Design review of the part built by this model. Coordinates are the model's own, in mm. A direction names the side the tool comes from. Round coordinates to 2 decimals unless told otherwise and drop trailing zeros. Order: outer loops, then holes, each group sorted by start corner. A loop starts at its lowest first (then second) coordinate and runs counter-clockwise, first axis right, second up.
from build123d import *

# Parameters (mm, degrees)
SKETCH_1_W          = 70
SKETCH_1_H          = 43
EXTRUDE_1_DEPTH     = 10.5
SKETCH_2_R          = 1.5
CUT_EXTRUDE_1_DEPTH = 15
SKETCH_3_W          = 41
SKETCH_3_H          = 20.2
CUT_EXTRUDE_2_DEPTH = 6
SKETCH_4_R          = 7
CUT_EXTRUDE_3_DEPTH = 8.5
SKETCH_6_W          = 39
SKETCH_6_H          = 20.2
CUT_EXTRUDE_4_DEPTH = 2.5
SKETCH_7_R          = 1.525
CUT_EXTRUDE_5_DEPTH = 5
SKETCH_9_W          = 55
SKETCH_9_H          = 1.8
CUT_EXTRUDE_6_DEPTH = 2
FILLET_1_R          = 8
SKETCH_10_R         = 7
SKETCH_10_R_2       = 1.5
SKETCH_10_R_3       = 1.525
CUT_EXTRUDE_7_DEPTH = 20
SKETCH_11_R         = 1.6
CUT_EXTRUDE_8_DEPTH = 1


with BuildPart() as part:
    # 草图1 → 凸台-拉伸1 (new body)
    with BuildSketch(Plane(origin=(0, 0, 0), x_dir=(1, 0, 0), z_dir=(0, 1, 0))):
        with Locations((0, 3.5)):
            Rectangle(SKETCH_1_W, SKETCH_1_H)
    extrude(amount=EXTRUDE_1_DEPTH)

    # 草图2 → 切除-拉伸1 (cut)
    with BuildSketch(Plane(origin=(0, 10.5, 0), x_dir=(1, 0, 0), z_dir=(0, 1, 0))):
        with Locations((15.1, 0)):
            Circle(SKETCH_2_R)
        with Locations((-15.1, 0)):
            Circle(SKETCH_2_R)
    extrude(amount=-CUT_EXTRUDE_1_DEPTH, mode=Mode.SUBTRACT)

    # 草图3 → 切除-拉伸2 (cut)
    with BuildSketch(Plane.XZ):
        with Locations((5.1, 0)):
            Rectangle(SKETCH_3_W, SKETCH_3_H)
    extrude(amount=-CUT_EXTRUDE_2_DEPTH, mode=Mode.SUBTRACT)

    # 草图4 → 切除-拉伸3 (cut)
    with BuildSketch(Plane.XZ.offset(-6)):
        with Locations((15.1, 0)):
            Circle(SKETCH_4_R)
    extrude(amount=-CUT_EXTRUDE_3_DEPTH, mode=Mode.SUBTRACT)

    # 草图6 → 切除-拉伸4 (cut)
    with BuildSketch(Plane.XZ.offset(-6)):
        with Locations((6.1, 0)):
            Rectangle(SKETCH_6_W, SKETCH_6_H)
    extrude(amount=-CUT_EXTRUDE_4_DEPTH, mode=Mode.SUBTRACT)

    # 草图7 → 切除-拉伸5 (cut)
    with BuildSketch(Plane.XZ):
        with Locations((29.2, 5)):
            Circle(SKETCH_7_R)
        with Locations((29.2, -5)):
            Circle(SKETCH_7_R)
        with Locations((-19, -5)):
            Circle(SKETCH_7_R)
        with Locations((-19, 5)):
            Circle(SKETCH_7_R)
    extrude(amount=-CUT_EXTRUDE_5_DEPTH, mode=Mode.SUBTRACT)

    # 草图9 → 切除-拉伸6 (cut)
    with BuildSketch(Plane.XZ):
        with Locations((5.1, 0)):
            Rectangle(SKETCH_9_W, SKETCH_9_H)
    extrude(amount=-CUT_EXTRUDE_6_DEPTH, mode=Mode.SUBTRACT)

    # 圆角1
    fillet_1_edges = [part.edges().sort_by_distance(p)[0] for p in [
        (-35, 5.25, -25),
        (35, 5.25, -25),
    ]]
    fillet(fillet_1_edges, radius=FILLET_1_R)

    # 草图10 → 切除-拉伸7 (cut)
    with BuildSketch(Plane(origin=(0, 10.5, 0), x_dir=(1, 0, 0), z_dir=(0, 1, 0))):
        with Locations((15.1, 0)):
            Circle(SKETCH_10_R)
        with Locations((-15.1, 0)):
            Circle(SKETCH_10_R_2)
        with Locations((-5.01238383, 20)):
            Circle(SKETCH_10_R_3)
        with Locations((5.01238383, 20)):
            Circle(SKETCH_10_R_3)
    extrude(amount=-CUT_EXTRUDE_7_DEPTH, mode=Mode.SUBTRACT)

    # 草图11 → 切除-拉伸8 (cut)
    with BuildSketch(Plane.XY.offset(18)):
        with Locations((0, 7.607443484)):
            Circle(SKETCH_11_R)
    extrude(amount=-CUT_EXTRUDE_8_DEPTH, mode=Mode.SUBTRACT)


solid = part.part
1) To check wall thickness, follow line 1 along X through (y, z) = (7, 0); line 2 along Z through (x, y) = (-19, 3.2) (3 decimals); line 3 along Z through (x, y) = (14.5, 5.25). State the ranges of each line that lie inside material, in increasing order.
Results:
line 1: x = -35 to -16.6, -13.6 to -13.4, 25.6 to 35
line 2: z = -25 to -6.525, -3.475 to 3.475, 6.525 to 18
line 3: z = -25 to -10.1, 10.1 to 18
2) For faces 4 (the face through (-19, 2, 0)), 5 (the face through (35, 5, 1)), list the 3-axis set-ups (+Z, -Z, +X, -X, +Y, -Y) from which the entire face can be reached by the end or side of a thin tool; tool diameter is ignored.
Results:
face 4: -Y
face 5: +Z, -Z, +X, +Y, -Y
3) Take a section at C-C on z = -5. Give the boundary of the cut face in (x, y) (3 decimals), plus the area to 3 significant figures.
Results:
outline: (-35, 0) - (-20.525, 0) - (-20.525, 5) - (-17.475, 5) - (-17.475, 0) - (-15.4, 0) - (-15.4, 6) - (-13.4, 6) - (-13.4, 8.5) - (10.201, 8.5) - (10.201, 10.5) - (-35, 10.5) - close; (19.999, 8.5) - (25.6, 8.5) - (25.6, 0) - (27.675, 0) - (27.675, 5) - (30.725, 5) - (30.725, 0) - (35, 0) - (35, 10.5) - (19.999, 10.5) - close
area: 341 mm2
4) Take a section at D-D on z = -20. Give the boundary of the cut face in (x, y), plus the area to 3 significant figures.
Results:
outline: (-34.42, 0) - (-6.54, 0) - (-6.54, 10.5) - (-34.42, 10.5) - close; (-3.49, 0) - (3.49, 0) - (3.49, 10.5) - (-3.49, 10.5) - close; (6.54, 0) - (34.42, 0) - (34.42, 10.5) - (6.54, 10.5) - close
area: 659 mm2
5) The part is to be moulded in two halves that separate along Y. For faces 1 (the face through (-16.3, 6.5, 0.9)), 2 (the face through (-0.347, 6.045, 17.507)), 3 (the face through (-14, 6, 2)), say which applies: released by +Y, released by -Y, zero draft, split by the parting line, or undercut.
Results:
face 1: zero draft
face 2: undercut
face 3: released by -Y
6) Clearance check with flat-ended pins moving along their axes: P1, Ø1.5, axis at x = 28.5, z = 5, coming from the -Y side; P2, Ø6, axis at x = 1, z = 3.5, coming from the -Y side; P3, Ø2.5, axis at x = -15.1, z = 0, coming from the -Y side. State where each tip first meets the part, or that it passes through.
Results:
P1: stops at y = 5
P2: stops at y = 8.5
P3: passes through
7) Take a section at A-A on y = 1.25. Give the boundary of the cut face in (x, z) (3 decimals), plus the area to 3 significant figures.
Results:
outline: (-35, -17) arc R8 ccw to (-27, -25) - (27, -25) arc R8 ccw to (35, -17) - (35, 18) - (-35, 18) - close; hole (-22.4, -0.9) - (-16.3, -0.9) arc R1.5 ccw to (-15.4, -1.47) - (-15.4, -10.1) - (25.6, -10.1) - (25.6, -0.9) - (32.6, -0.9) - (32.6, 0.9) - (25.6, 0.9) - (25.6, 10.1) - (-15.4, 10.1) - (-15.4, 1.47) arc R1.5 ccw to (-16.3, 0.9) - (-22.4, 0.9) - close; hole circle Ø3.05 at (-19, -5); hole circle Ø3.05 at (-19, 5); hole circle Ø3.05 at (-5.012, -20); hole circle Ø3.05 at (5.012, -20); hole circle Ø3.05 at (29.2, -5); hole circle Ø3.05 at (29.2, 5)
area: 2,080 mm2
8) Take a section at B-B on x = -19. Give the boundary of the cut face in (y, z) (3 decimals).
Results:
outline: (0, -25) - (10.5, -25) - (10.5, 18) - (0, 18) - (0, 6.525) - (5, 6.525) - (5, 3.475) - (0, 3.475) - (0, 0.9) - (2, 0.9) - (2, -0.9) - (0, -0.9) - (0, -3.475) - (5, -3.475) - (5, -6.525) - (0, -6.525) - close
